from build123d import *

# Parameters (mm, degrees)
F0_R            = 11
F1_DEPTH        = 4
F3_DEPTH        = 4.001
F3_COPIES_COUNT = 12
F5_R            = 3.2
F6_DEPTH        = 3
F7_W            = 3.6
F7_H            = 3.6
F8_DEPTH        = 7.001


# Not quite as in the source:
# - a pattern or mirror of a feature is missing from the dataset's text; its kind, count and spacing are read off the source's solid


with BuildPart() as f1:
    # F0 (on Top) → F1 (new body)
    with BuildSketch(Plane.XY):
        Circle(F0_R)
    extrude(amount=F1_DEPTH)

    # F2 (on face) → F3 (cut, through all)
    with BuildSketch(Plane.XY.offset(4)):
        with BuildLine():
            Line((0, 11), (0, 7))
            ThreePointArc((0, 7), (0.1221668451, 6.9989338661), (0.2442964769, 6.9957357891))
            Line((0.2442964769, 6.9957357891), (2.8470094961, 10.6251840892))
            ThreePointArc((2.8470094961, 10.6251840892), (1.4357881144, 10.9058934751), (0, 11))
        make_face()
        with BuildLine():
            ThreePointArc((-0.2442964769, 6.9957357891), (-0.1221668451, 6.9989338661), (0, 7))
            Line((0, 7), (0, 11))
            ThreePointArc((0, 11), (-1.2452353514, 10.9292904124), (-2.4744615978, 10.7180707126))
            Line((-2.4744615978, 10.7180707126), (-0.2442964769, 6.9957357891))
        make_face()
    f3 = extrude(amount=-F3_DEPTH, mode=Mode.SUBTRACT)

    # F3_copies: F3 ×12 about axis
    f3_copies_axis = Axis((0, 0, 0), (0, 0, 1))
    for i in range(1, F3_COPIES_COUNT):
        add(f3.rotate(f3_copies_axis, i * 360 / F3_COPIES_COUNT), mode=Mode.SUBTRACT)

    # F5 (on face) → F6 (join)
    with BuildSketch(Plane(origin=(0, 0, 0), x_dir=(1, 0, 0), z_dir=(0, 0, -1))):
        Circle(F5_R)
    extrude(amount=F6_DEPTH)

    # F7 (on face) → F8 (cut, through all)
    with BuildSketch(Plane(origin=(0, 0, -3), x_dir=(1, 0, 0), z_dir=(0, 0, -1))):
        Rectangle(F7_W, F7_H)
    extrude(amount=-F8_DEPTH, mode=Mode.SUBTRACT)


solid = f1.part
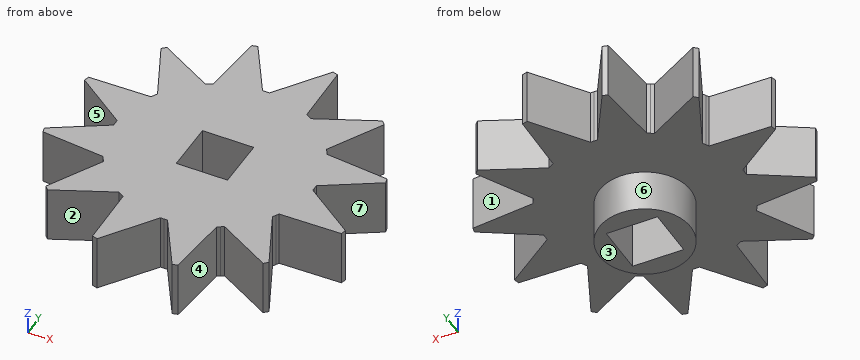
Here's how the part is built. I have some questions about the finished solid (model axes, mm). Face numbers are marked on the shaded views. A direction names the side the tool comes from. Coordinates: 2 decimals unless noted, no trailing zeros. Write each loop counter-clockwise with the first axis right and the second up, starting at its lowest first coordinate (ties: lowest second). Pieces come first, ordered by that corner, then holes.
1) I'm going to push flat-ended pins straight in: pin 1 (4 mm diameter, centred on x = 3.5, z = -1.5, fed in from +Y); pin 2 (1.8 mm diameter, centred on x = -0.5, z = 2, fed in from +Y); pin 3 (4 mm diameter, centred on x = 6.5, y = -5.5, fed in from -Z); pin 4 (10.5 mm diameter, centred on x = -2, y = 4.5, fed in from -Z). Where does each tip first touch, or does it pass through?
Filled in:
pin 1: stops at y = 10.63
pin 2: stops at y = 8.92
pin 3: stops at z = 0
pin 4: stops at z = -3
2) Which directions (+Z, -Z, +X, -X, +Y, -Y) give clear straight access to the entire face, cutting with the end or side of a thin tool? Please do the marked faces 4, 5, 6 and 7.
Filled in:
face 4: +Z, -Z, -Y
face 5: +Z, -Z, -X
face 6: -Z
face 7: +Z, -Z, +X
3) If we section it at B-B (z = -1.5): List the corners of the cut face in (x, y) for me, plus the area to 3 significant figures.
Filled in:
outline: circle Ø6.4 at (0, 0); hole (-1.8, -1.8) - (1.8, -1.8) - (1.8, 1.8) - (-1.8, 1.8) - close
area: 19.2 mm2
4) If I drill on line 1 (Y direction, x = 0, z = 2.75); line 2 (X direction, y = -6.25, z = 2.5); line 3 (Z direction, x = -7.25, y = -2.5), over which ranges is the centre line in solid material (lowest first)?
Filled in:
line 1: y = -7 to -1.8, 1.8 to 7
line 2: x = -7.35 to -4.4, -3.29 to 3.28, 4.27 to 7.09
line 3: z = 0 to 4
5) If we section it at D-D (x = -5): List the corners of the cut face in (y, z) for me, plus the area to 3 significant figures.
Filled in:
outline: (-6.52, 0) - (6.65, 0) - (6.65, 4) - (-6.52, 4) - close
area: 52.7 mm2
6) If we section it at A-A (x = -1): List the corners of the cut face in (y, z) for me.
Filled in:
outline: (-8.05, 0) - (-3.04, 0) - (-3.04, -3) - (-1.8, -3) - (-1.8, 4) - (-8.05, 4) - close; (1.8, -3) - (3.04, -3) - (3.04, 0) - (8.26, 0) - (8.26, 4) - (1.8, 4) - close
7) If we section it at C-C (y = 9.75): List the corners of the cut face in (x, z) for me.
Filled in:
outline: (-2.93, 0) - (-1.89, 0) - (-1.89, 4) - (-2.93, 4) - close; (2.22, 0) - (3.23, 0) - (3.23, 4) - (2.22, 4) - close
8) Thinking about a two-plate mould opening in Y: for the marked faces 1, 2 and 3, which applies, +Y half, -Y half, draft (parallel to the pull), parting line (faces both ways), or undercut?
Filled in:
face 1: undercut
face 2: -Y half
face 3: draft
